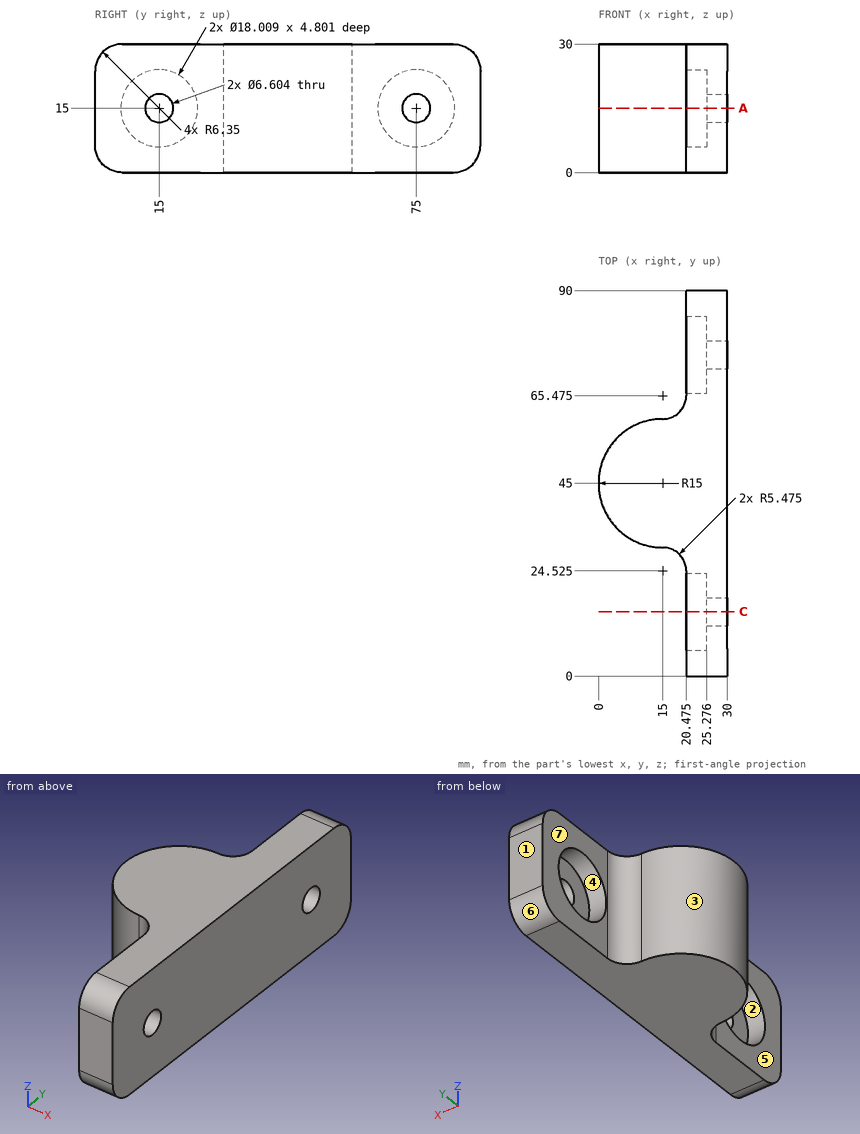
Can you work these out from the drawing? Everything is in mm from the part's minimum corner. A direction names the side the tool comes from. Round coordinates to 2 decimals unless told otherwise and drop trailing zeros. Loops run counter-clockwise (first coordinate to the right, second up) from the corner with the lowest first, then second, coordinate; pieces in that order, holes last. Notation, with made-up numbers: (57.25, 25) - (114.25, 25) arc R10 cw to (114.25, 44) - close; hole circle Ø11 at (-35, -40). An arc over 180 degrees is marked (long way). One line per question, with ' | ' between items. Start each with the question number.
Q1. I want a section at A-A (z = 15). State how many separate pieces and enclosed holes the cut face has, then the cut area to 3 significant figures.
Q2. I want a section at C-C (y = 15). Write out the boundary of the cut face in (x, z) (1 decimal).
Q3. Will these pins go through, and if not, where does the flat tip stop? pin 1 (3 mm diameter, centred on x = 8.5, z = 16, fed in from +Y); pin 2 (6 mm diameter, centred on y = 15, z = 15, fed in from -X); pin 3 (5.5 mm diameter, centred on y = 73, z = 13.5, fed in from -X); pin 4 (1 mm diameter, centred on x = 6, z = 23.5, fed in from +Y).
Q4. We'd pull the mould along Y, two halves only. Please class the marked faces 1, 2, 3 and 4: +Y half, -Y half, draft (parallel to the pull), parting line (faces both ways), or undercut.
Q5. Please list where these lines run through material, in increasing order: line 1 (Y direction, x = 27.35, z = 15); line 2 (Y direction, x = 22.5, z = 10.25); line 3 (Z direction, x = 28.9, y = 75). Write a range as [from, to].
Q6. For the marked faces 5, 6 and 7, which set-ups out of +Z, -Z, +X, -X, +Y, -Y let a thin tool reach every point of the face, with its end or its side?
Response values:
1) separate pieces: 3 | enclosed holes: 0 | area: 1,150 mm²
2) outline: (20.5, 0) - (30, 0) - (30, 11.7) - (25.3, 11.7) - (25.3, 6) - (20.5, 6) - close; (20.5, 24) - (25.3, 24) - (25.3, 18.3) - (30, 18.3) - (30, 30) - (20.5, 30) - close
3) pin 1: stops at y = 59.14 | pin 2: passes through | pin 3: stops at x = 25.28 | pin 4: stops at y = 57.36
4) face 1: +Y half | face 2: undercut | face 3: parting line | face 4: undercut
5) line 1: y = [0, 11.7], [18.3, 71.7], [78.3, 90] | line 2: y = [0, 7.35], [22.65, 67.35], [82.65, 90] | line 3: z = [0, 11.7], [18.3, 30]
6) face 5: +Z, -Z, -X, -Y | face 6: -Z, +X, -X, +Y | face 7: +Z, -Z, -X, +Y
